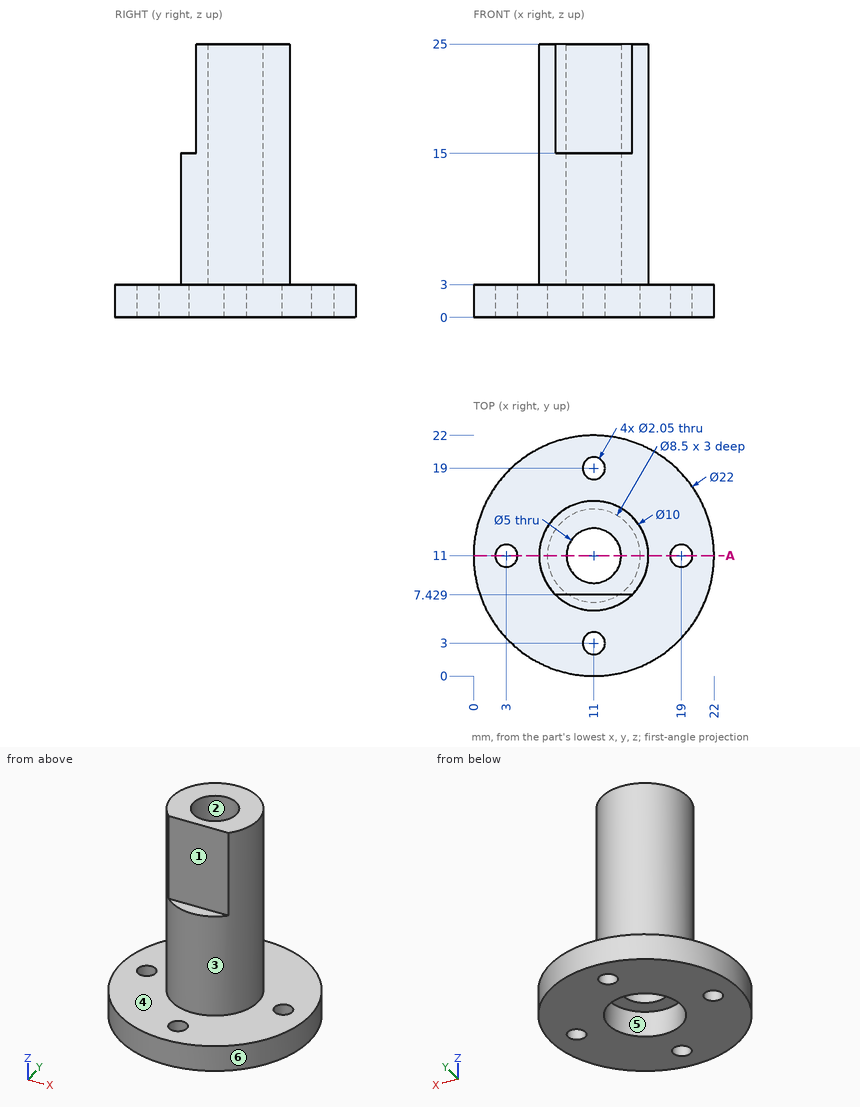
Verification items for this drawing (mm, ordinates from the low corner). A direction names the side the tool comes from. Give positions to 0.01 mm unless a question says otherwise; leave off trailing zeros. Write item = value, one per line. Start each with the question number.
Q1. Depth check by flat-ended pin: P1, Ø5.5, axis at x = 12.5, z = 20, coming from the -Y side; P2, Ø1.5, axis at x = 4.5, z = 4, coming from the +Y side; P3, Ø1.5, axis at y = 10.5, z = 7.5, coming from the +X side; P4, Ø1.5, axis at x = 6.5, z = 14.5, coming from the +Y side. Enter the tip coordinate at first touch or a pass-through.
Q2. Thickness scan on line 1 (Z direction, x = 3.75, y = 5.25); line 2 (X direction, y = 11, z = 11.5); line 3 (Z direction, x = 14, y = 13). Record the ranges inside material, lowest first.
Q3. Tool access check on the marked faces 4, 5 and 6. Record the directions out of +Z, -Z, +X, -X, +Y, -Y that give a thin tool (end or side, any length) a straight path to the whole face; none if there is none.
Q4. Cross-section at A-A, the plane y = 11. State how many separate pieces and enclosed holes the cut face has, and give its area (3 significant figures).
Q5. Mould release check, pull along Y, two halves, no side actions. Record for the marked faces 1, 2 and 3: released by +Y, released by -Y, zero draft, split by the parting line, or undercut.
Answer key:
q1.P1 = 7.43
q1.P2 = through
q1.P3 = 16
q1.P4 = 14.31
q2.line_1 = 0 to 3
q2.line_2 = 6 to 8.5, 13.5 to 16
q2.line_3 = 3 to 25
q3.face_4 = +Z
q3.face_5 = -Z
q3.face_6 = +Z, -Z
q4.separate_pieces = 4
q4.enclosed_holes = 0
q4.area = 138 mm^2
q5.face_1 = released by -Y
q5.face_2 = undercut
q5.face_3 = split by the parting line
